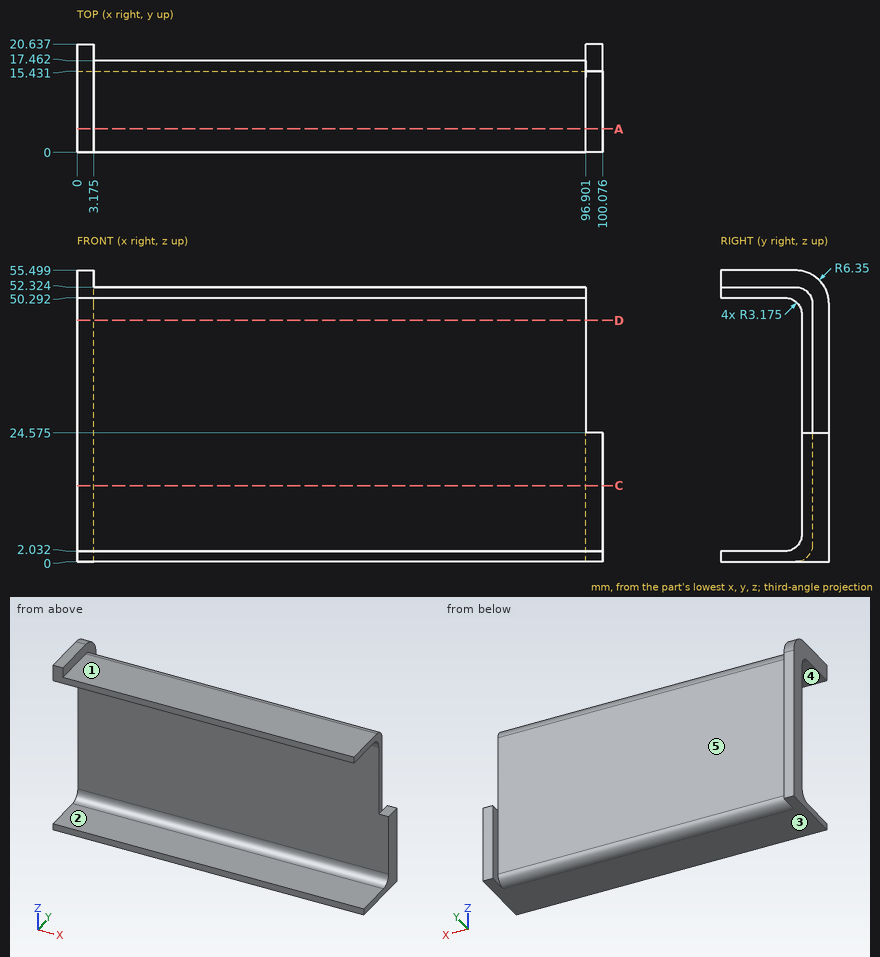
Answer from the drawing. Dimensions are ordinates in mm from the lowest x, y and z of the part. A direction names the side the tool comes from. Give positions to 0.01 mm unless a question says otherwise; leave off trailing zeros. Order: outer loops, then holes, each group sorted by start corner. A loop starts at its lowest first (then second) coordinate and runs counter-clockwise, first axis right, second up. Notation, with made-up numbers: (-27, 72.25) - (-12, 72.25) arc R21 cw to (-12, 97.25) - close; hole circle Ø9 at (77.25, 27). An arc over 180 degrees is marked (long way). One line per item, written item: value. Start each with the question number.
1. Each of these flat-tipped pins is pushed along its axis until it touches: pin 1 Ø6 at (x, y) = (42, 4) entering from +Z; pin 2 Ø3 at (x, z) = (51, 38.5) entering from -Y; pin 3 Ø10 at (x, z) = (89.5, 46) entering from +Y; pin 4 Ø10 at (x, y) = (54, 7) entering from -Z. Where does it stop, or does it pass through?
2. For a pull along Z with two mould halves and no side action, classify the marked faces 1, 2 and 3 as released by +Z, released by -Z, zero draft, split by the parting line, or undercut.
3. Section A-A, the plane y = 4.5 is taken. Write down the section's boundary in (x, z) (1 decimal).
4. Which of the six approach directions +Z, -Z, +X, -X, +Y, -Y give full straight-line access (tool end or side, diameter ignored) to the marked faces 4 and 5?
5. Section C-C, the plane z = 14.5 is taken. Write down the section's boundary in (x, y) (1 decimal).
6. Consider line 1 (Z direction, x = 72, y = 9.5) (1 decimal); line 2 (Y direction, x = 78.5, z = 42); line 3 (X direction, y = 19.5, z = 29.5) (1 decimal). Determine where each line is inside the solid, lowest interval first.
7. Section D-D, the plane z = 46 is taken. Write down the section's boundary in (x, y) (1 decimal).
Filled sheet:
1. pin 1: z = 52.32
1. pin 2: y = 15.43
1. pin 3: y = 17.46
1. pin 4: z = 0
2. face 1: released by +Z
2. face 2: undercut
2. face 3: released by -Z
3. outline: (0, 0) - (100.1, 0) - (100.1, 2) - (0, 2) - close; (0, 50.3) - (96.9, 50.3) - (96.9, 52.3) - (3.2, 52.3) - (3.2, 55.5) - (0, 55.5) - close
4. face 4: +X, -X, -Y
4. face 5: +Z, -Z, +Y
5. outline: (0, 15.4) - (100.1, 15.4) - (100.1, 20.6) - (96.9, 20.6) - (96.9, 17.5) - (3.2, 17.5) - (3.2, 20.6) - (0, 20.6) - close
6. line 1: 0 to 2, 50.3 to 52.3
6. line 2: 15.43 to 17.46
6. line 3: 0 to 3.2
7. outline: (0, 15.4) - (96.9, 15.4) - (96.9, 17.5) - (3.2, 17.5) - (3.2, 20.6) - (0, 20.6) - close
